Part model, mm, in its own coordinate system. Coordinates: 2 decimals unless noted, no trailing zeros. Order: outer loops, then holes, each group sorted by start corner. A loop starts at its lowest first (then second) coordinate and runs counter-clockwise, first axis right, second up. Notation, with made-up numbers: M 81,6 L 89,6 A12 cw 89,15 Z; hole C 41.5,-31.5 d4. An arc over 180 degrees is marked long. Answer in a Markdown table with one row per item. Add a question column.
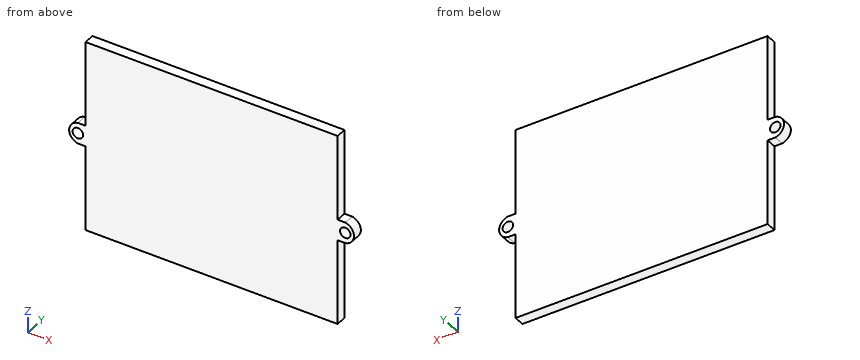
Autodesk Inventor part; units mm, degrees
ref_plane "YZ Plane" through (0, 0, 0) normal (1, 0, 0) x (0, 1, 0)
ref_plane "XZ Plane" through (0, 0, 0) normal (0, 1, 0) x (-1, 0, 0)
ref_plane "XY Plane" through (0, 0, 0) normal (0, 0, 1) x (1, 0, 0)
sketch "Esboço1" plane through (0, 0, 0) normal (0, 1, 0) x (-1, 0, 0)
  line L0 (35.5878, 45.6911) -> (-44.4122, 45.6911)
  line L1 (-44.4122, 45.6911) -> (-44.4122, -14.3089)
  line L2 (-44.4122, -14.3089) -> (35.5878, -14.3089)
  line L3 (35.5878, -14.3089) -> (35.5878, 45.6911)
  line L4 (35.5878, 45.6911) -> (35.5878, -14.3089)
  line L5 (45.5878, 15.6911) -> (-44.4122, 15.6911)
  line L6 (-4.4122, 85.6911) -> (-4.4122, -84.3089)
  line L7 (-44.4122, -14.3089) -> (-44.4122, 45.6911)
  line L8 (37.5878, 47.6911) -> (-46.4122, 47.6911)
  line L9 (-46.4122, -16.3089) -> (37.5878, -16.3089)
  circle A0 centre (40.1473, 15.6911) radius 1.75
  line L10 (40.1473, 19.1911) -> (37.5878, 19.1911)
  line L11 (37.5878, 12.1911) -> (40.1473, 12.1911)
  arc A1 (40.1473, 12.1911) -> (40.1473, 19.1911) centre (39.4884, 15.6911) ccw
  line L12 (37.5878, -16.3089) -> (37.5878, 12.1911)
  line L13 (37.5878, 19.1911) -> (37.5878, 47.6911)
  line L14 (-48.9716, 19.1911) -> (-46.4122, 19.1911)
  line L15 (-46.4122, 12.1911) -> (-48.9716, 12.1911)
  circle A2 centre (-48.9716, 15.6911) radius 1.75
  arc A3 (-48.9716, 19.1911) -> (-48.9716, 12.1911) centre (-48.3127, 15.6911) ccw
  line L16 (-46.4122, 47.6911) -> (-46.4122, 19.1911)
  line L17 (-46.4122, 12.1911) -> (-46.4122, -16.3089)
  point P0 (0, 0)
  point P1 (0.5878, 15.6911)
  point P2 (-4.4122, -16.3089)
  dimension "d2" = 60
  dimension "d3" = 30
  dimension "d4" = 80
  dimension "d5" = 64
  dimension "d6" = 32
  dimension "d7" = 3.5
  dimension "d8" = 3.5
extrude "Extrusão1" add sketch "Esboço1" along normal blind 3.5 contours L3 L5 L6 L0 | L0 L6 L8 L13 L10 A1 L5 A0 L3 | L6 L5 L1 L0 | L0 L1 L2 L6 L9 L17 L15 A3 L14 L16 L8 | L5 A0 A1 L11 L12 L9 L6 L2 L3 | L3 L2 L6 L5 | L6 L2 L1 L5
properties part number "tampa_pilha"
(1) Wall check: line 1 (X direction, y = 0.8, z = 35.5). Give the ranges that are in metal, low to high.
(2) Slice it at A-A (y = 2.45). List the corners of the cut face in (x, z), and give its area (3 significant figures).
(3) Drop flat-ended pins along their axis: P1, Ø1, axis at y = 2.5, z = -3.5, coming from the +X side; P2, Ø1.3, axis at x = -39, y = 2, coming from the +Z side; P3, Ø2, axis at x = -39, y = 1.5, coming from the -Z side. Give the stop position or say it passes through.
(4) Slice it at B-B (z = 4.5). List the corners of the cut face in (x, y), and give its area (3 significant figures).
Computed:
| question | item | result |
|---|---|---|
| 1 | line 1 | x = -37.59 to 46.41 |
| 2 | outline | M -40.15,12.19 L -37.59,12.19 L -37.59,-16.31 L 46.41,-16.31 L 46.41,12.19 L 48.97,12.19 A3.56 ccw 48.97,19.19 L 46.41,19.19 L 46.41,47.69 L -37.59,47.69 L -37.59,19.19 L -40.15,19.19 A3.56 ccw Z; hole C -40.15,15.69 d3.5; hole C 48.97,15.69 d3.5 |
| 2 | area | 5,420 mm^2 |
| 3 | P1 | stops at x = 46.41 |
| 3 | P2 | stops at z = 19.19 |
| 3 | P3 | stops at z = 12.19 |
| 4 | outline | M -37.59,0 L 46.41,0 L 46.41,3.5 L -37.59,3.5 Z |
| 4 | area | 294 mm^2 |
